Work out the finished part from the listing and answer in its coordinate system (mm). Face numbers are marked on the shaded views. A direction names the side the tool comes from. Coordinates: 2 decimals unless noted, no trailing zeros. Order: outer loops, then holes, each group sorted by start corner. A loop starts at its lowest first (then second) coordinate and runs counter-clockwise, first axis right, second up. Notation, with made-up numbers: M -36,-14.5 L 1,-14.5 A34 cw 1,23.5 Z; hole C 82.5,25.25 d9. An arc over 180 degrees is marked long. Write item = value, one per line. Start each with the question number.
Q1. A tool of negligible diameter and unlimited length cuts with its end or side. For the marked faces 4, 5, 6, 7 and 8, from which of +Z, -Z, +X, -X, +Y, -Y can it reach the whole face along a straight path? Write none if from no direction.
Q2. Each of these flat-tipped pins is pushed along its axis until it touches: P1, Ø5.5, axis at y = 5.5, z = 10, coming from the +X side; P2, Ø10.5, axis at x = -10, z = 16, coming from the -Y side; P3, Ø1, axis at x = 25, z = 19, coming from the -Y side. Where does it stop, or does it pass through?
Q3. Straight lines are drawn through the part: line 1 along Z through (x, y) = (-10, 13.75); line 2 along Y through (x, z) = (33, 16.5); line 3 along Y through (x, z) = (27, 21). For each, find the intervals that lie inside material, in ascending order.
Q4. Find section C-C on y = 8. Give the vertices of the cut face in (x, z).
Q5. Find section B-B on x = 10. Give the vertices of the cut face in (y, z).
Q6. Find section A-A on z = 6. Give the vertices of the cut face in (x, y).
Q7. Determine the mould class of the marked faces 1, 2 and 3 for opening direction X: released by +X, released by -X, zero draft, split by the parting line, or undercut.
Q8. Find section D-D on x = -10. Give the vertices of the cut face in (y, z).
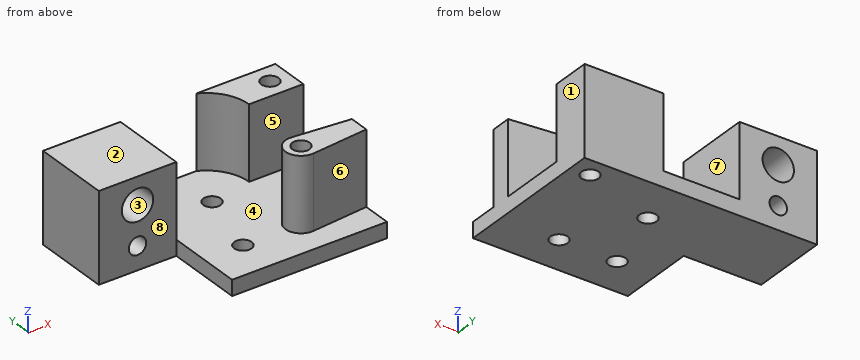
```python
from build123d import *

# Parameters (mm, degrees)
SKETCH_R        = 2.25
PAD_DEPTH       = 23
POCKET_DEPTH    = 19
SKETCH002_R     = 4.05
SKETCH002_R_2   = 2.25
POCKET001_DEPTH = 20.001


with BuildPart() as part:
    # Sketch → Pad (new body)
    with BuildSketch(Plane.XY):
        Polygon((0, -20), (40, -20), (40, 20), (-20, 20), (-20, 0), (0, 0), align=None)
        with Locations((15, 8)):
            Circle(SKETCH_R, mode=Mode.SUBTRACT)
        with Locations((10, -10)):
            Circle(SKETCH_R, mode=Mode.SUBTRACT)
        with Locations((25, -10)):
            Circle(SKETCH_R, mode=Mode.SUBTRACT)
        with Locations((35, 15)):
            Circle(SKETCH_R, mode=Mode.SUBTRACT)
    extrude(amount=PAD_DEPTH)

    # Sketch001 → Pocket (cut)
    with BuildSketch(Plane.XY.offset(23)):
        with BuildLine():
            Line((46, 10), (26, 10))
            ThreePointArc((26, 10), (22.778175, 17.778175), (15, 21))
            Line((15, 21), (0, 21))
            Line((0, 21), (0, -23))
            Line((0, -23), (46, -23))
            Line((46, -23), (46, -12))
            Line((25.382674, -13.981653), (46, -12))
            ThreePointArc((25.382674, -6.018347), (21, -10), (25.382674, -13.981653))
            Line((25.382674, -6.018347), (46, -8))
            Line((46, -8), (46, 10))
        make_face()
    extrude(amount=-POCKET_DEPTH, mode=Mode.SUBTRACT)

    # Sketch002 → Pocket001 (cut, through all)
    with BuildSketch(Plane.XZ):
        with Locations((-10, 16)):
            Circle(SKETCH002_R)
        with Locations((-10, 6)):
            Circle(SKETCH002_R_2)
    extrude(amount=-POCKET001_DEPTH, mode=Mode.SUBTRACT)


solid = part.part
```
Findings below:
q1.face_4 = +Z
q1.face_5 = +Z, +X
q1.face_6 = +Z, +X, -Y
q1.face_7 = +Z, +Y, -Y
q1.face_8 = +Z, -Z, -X, -Y
q2.P1 = 0
q2.P2 = 0
q2.P3 = -14
q3.line_1 = 0 to 3.75, 8.25 to 11.95, 20.05 to 23
q3.line_2 = -13.25 to -6.75, 10 to 13.97, 16.03 to 20
q3.line_3 = -13.83 to -11.03, -8.97 to -6.17, 10 to 20
q4.outline = M -20,0 L 12.75,0 L 12.75,4 L 0,4 L 0,23 L -20,23 Z; M 17.25,0 L 40,0 L 40,4 L 17.25,4 Z; hole C -10,16 d8.1; hole C -10,6 d4.5
q5.outline = M -20,0 L -12.25,0 L -12.25,4 L -20,4 Z; M -7.75,0 L 20,0 L 20,4 L -7.75,4 Z
q6.outline = M -20,0 L -12.25,0 L -12.25,20 L -20,20 Z; M -7.75,0 L 0,0 L 0,20 L -7.75,20 Z; M 19.58,20 A11 cw 26,10 L 40,10 L 40,20 Z; M 25.38,-13.98 L 40,-12.58 L 40,-7.42 L 25.38,-6.02 A4 ccw long Z; hole C 25,-10 d4.5; hole C 35,15 d4.5
q7.face_1 = released by +X
q7.face_2 = zero draft
q7.face_3 = undercut
q8.outline = M 0,0 L 20,0 L 20,3.75 L 0,3.75 Z; M 0,8.25 L 20,8.25 L 20,11.95 L 0,11.95 Z; M 0,20.05 L 20,20.05 L 20,23 L 0,23 Z
